Source: CAD feature listing. Evaluate the final solid. Frame: model axes, mm. Coordinates: 2 decimals unless noted, no trailing zeros. Write each loop counter-clockwise with the first axis right and the second up, starting at its lowest first coordinate (ties: lowest second). Pieces come first, ordered by that corner, then holes. Notation, with made-up numbers: (66, -19.75) - (88, -19.75) arc R7 ccw to (88, -12.75) - close; hole circle Ø3 at (61.25, 24). An arc over 180 degrees is marked (long way). One line per item, written item: value.
from build123d import *

# Parameters (mm, degrees)
SKETCH1_W           = 596.9
SKETCH1_H           = 355.6
BOSS_EXTRUDE1_DEPTH = 9.525
CHAMFER1_SIZE       = 19.05


with BuildPart() as part:
    # Sketch1 → Boss-Extrude1 (new, symmetric)
    with BuildSketch(Plane(origin=(0, 0, 0), x_dir=(1, 0, 0), z_dir=(0, 1, 0))):
        Rectangle(SKETCH1_W, SKETCH1_H)
    extrude(amount=BOSS_EXTRUDE1_DEPTH, both=True)

    # Chamfer1
    chamfer1_edges = [part.edges().sort_by_distance(p)[0] for p in [
        (298.45, -9.525, 0),
        (-298.45, -9.525, 0),
    ]]
    chamfer(chamfer1_edges, length=CHAMFER1_SIZE - 0.0001)  # a hair under: the kernel refuses the full size


solid = part.part
1) Contact query for flat-ended pins moving along their axis: P1, Ø4, axis at y = 6, z = -71, coming from the +X side; P2, Ø5, axis at y = 3, z = 34.5, coming from the +X side; P3, Ø8, axis at y = 2.5, z = -27, coming from the +X side. Output: stop coordinate, or through.
Values found:
P1: x = 296.93
P2: x = 294.43
P3: x = 295.43
2) Section query B-B on y = -4.5. Output: boundary loops of the cut face in (x, z).
Values found:
outline: (-284.43, -177.8) - (284.43, -177.8) - (284.43, 177.8) - (-284.43, 177.8) - close
3) Material intervals for line 1 (X direction, y = 6.5, z = -136); line 2 (X direction, y = -8.5, z = -121.5), sorted ascending.
Values found:
line 1: -295.43 to 295.43
line 2: -280.43 to 280.43
